```python
from build123d import *

# Parameters (mm, degrees)
SKETCH_2_R          = 2
SKETCH_2_R_2        = 5.5
SKETCH_2_R_3        = 2.5
EXTRUDE_1_DEPTH     = 1.5
SKETCH_3_R          = 2.5
CUT_EXTRUDE_1_DEPTH = 10


with BuildPart() as part:
    # 草图2 → 凸台-拉伸1 (new, symmetric)
    with BuildSketch(Plane.XY):
        with BuildLine():
            Line((120, 0), (207, 0))
            Line((207, 0), (207, 33.215924565))
            Line((207, 33.215924565), (208.99932908, 33.215924565))
            Line((208.99932908, 33.215924565), (208.99932908, 0))
            Line((208.99932908, 0), (250, 0))
            Line((250, 0), (250, 40))
            ThreePointArc((250, 40), (247.071067812, 47.071067812), (240, 50))
            Line((240, 50), (10, 50))
            ThreePointArc((10, 50), (2.928932188, 47.071067812), (0, 40))
            Line((0, 40), (0, 0))
            Line((0, 0), (30, 0))
            Line((30, 0), (120, 0))
        make_face()
        with Locations((10, 45)):
            Circle(SKETCH_2_R, mode=Mode.SUBTRACT)
        with Locations((10, 35)):
            Circle(SKETCH_2_R, mode=Mode.SUBTRACT)
        with Locations((60, 45)):
            Circle(SKETCH_2_R, mode=Mode.SUBTRACT)
        with Locations((60, 35)):
            Circle(SKETCH_2_R, mode=Mode.SUBTRACT)
        with Locations((25, 40)):
            Circle(SKETCH_2_R_2, mode=Mode.SUBTRACT)
        with Locations((6.5, 16.5)):
            Circle(SKETCH_2_R_3, mode=Mode.SUBTRACT)
        with Locations((23.5, 16.5)):
            Circle(SKETCH_2_R_3, mode=Mode.SUBTRACT)
        with Locations((220.5, 16.5)):
            Circle(SKETCH_2_R_3, mode=Mode.SUBTRACT)
        with Locations((237.5, 16.5)):
            Circle(SKETCH_2_R_3, mode=Mode.SUBTRACT)
    extrude(amount=EXTRUDE_1_DEPTH, both=True)

    # 草图3 → 切除-拉伸1 (cut)
    with BuildSketch(Plane.XY.offset(1.5)):
        with Locations((192, 25)):
            Circle(SKETCH_3_R)
        with Locations((192, 8)):
            Circle(SKETCH_3_R)
    extrude(amount=-CUT_EXTRUDE_1_DEPTH, mode=Mode.SUBTRACT)


solid = part.part
```
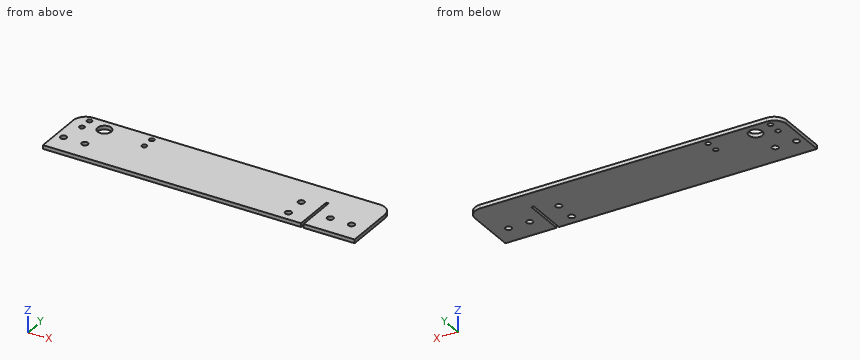
Build history of the part. All positions in model axes, mm. Coordinates: 2 decimals unless noted, no trailing zeros. Write each loop counter-clockwise with the first axis right and the second up, starting at its lowest first coordinate (ties: lowest second). Pieces come first, ordered by that corner, then holes.
1. Band-saw the part on C-C, the plane z = -0.65. Give the number of separate pieces and of enclosed holes in the cut face, and give its area (3 significant figures).
Answer block:
separate pieces: 1
enclosed holes: 11
area: 12,100 mm2
2. Band-saw the part on A-A, the plane y = 8. Give the cut face in (x, z).
Answer block:
outline: (0, -1.5) - (189.5, -1.5) - (189.5, 1.5) - (0, 1.5) - close; (194.5, -1.5) - (207, -1.5) - (207, 1.5) - (194.5, 1.5) - close; (209, -1.5) - (250, -1.5) - (250, 1.5) - (209, 1.5) - close
3. Drop a flat-ended pin along its axis: pin 1 (1 mm diameter, centred on x = 208, z = 0, fed in from -Y). Give the stop position or say it passes through.
Answer block:
pin 1: stops at y = 33.22
4. Band-saw the part on B-B, the plane x = 192. Give the cut face in (y, z).
Answer block:
outline: (0, -1.5) - (5.5, -1.5) - (5.5, 1.5) - (0, 1.5) - close; (10.5, -1.5) - (22.5, -1.5) - (22.5, 1.5) - (10.5, 1.5) - close; (27.5, -1.5) - (50, -1.5) - (50, 1.5) - (27.5, 1.5) - close
5. Drill centre lines: probe 1 along X at (y, z) = (24.5, -1.15); probe 2 along X at (y, z) = (31, 1.1); probe 3 along Y at (x, z) = (10, -0.1). Where is each one in solid material? Low to high.
Answer block:
probe 1: x = 0 to 189.55, 194.45 to 207, 209 to 250
probe 2: x = 0 to 207, 209 to 250
probe 3: y = 0 to 33, 37 to 43, 47 to 50
